Autodesk Inventor part; units mm, degrees
ref_plane "YZ Plane" through (0, 0, 0) normal (1, 0, 0) x (0, 1, 0)
ref_plane "XZ Plane" through (0, 0, 0) normal (0, 1, 0) x (-1, 0, 0)
ref_plane "XY Plane" through (0, 0, 0) normal (0, 0, 1) x (1, 0, 0)
sketch "Эскиз1" plane through (0, 0, 0) normal (0, 0, 1) x (1, 0, 0)
  circle A0 centre (0, 0) radius 40
  circle A1 centre (35, 35) radius 2
  circle A2 centre (-35, 35) radius 2
  circle A3 centre (-35, -35) radius 2
  circle A4 centre (35, -35) radius 2
  line L0 (72.777, 200) -> (-80, 200)
  line L1 (-80, 200) -> (-80, -200)
  line L2 (-80, -200) -> (72.777, -200)
  line L3 (72.777, -200) -> (72.777, 200)
  point P0 (0, 0)
  dimension "d0" = 400
  dimension "d1" = 200
  dimension "d2" = 80
extrude "Выдавливание1" add sketch "Эскиз1" along normal blind 4
sketch "Эскиз3" plane through (0, 0, 4) normal (0, 0, 1) x (1, 0, 0)
  line L0 (72.777, 200) -> (62.777, 200)
  line L1 (62.777, 200) -> (62.777, 196)
  line L2 (62.777, 196) -> (72.777, 196)
  line L3 (72.777, 196) -> (72.777, 200)
  line L4 (72.777, 200) -> (-80, 200)
  line L5 (52.777, 200) -> (42.777, 200)
  line L6 (42.777, 200) -> (42.777, 196)
  line L7 (42.777, 196) -> (52.777, 196)
  line L8 (52.777, 196) -> (52.777, 200)
  line L9 (32.777, 200) -> (22.777, 200)
  line L10 (22.777, 200) -> (22.777, 196)
  line L11 (22.777, 196) -> (32.777, 196)
  line L12 (32.777, 196) -> (32.777, 200)
  line L13 (12.777, 200) -> (2.777, 200)
  line L14 (2.777, 200) -> (2.777, 196)
  line L15 (2.777, 196) -> (12.777, 196)
  line L16 (12.777, 196) -> (12.777, 200)
  line L17 (-7.223, 200) -> (-17.223, 200)
  line L18 (-17.223, 200) -> (-17.223, 196)
  line L19 (-17.223, 196) -> (-7.223, 196)
  line L20 (-7.223, 196) -> (-7.223, 200)
  line L21 (-27.223, 200) -> (-37.223, 200)
  line L22 (-37.223, 200) -> (-37.223, 196)
  line L23 (-37.223, 196) -> (-27.223, 196)
  line L24 (-27.223, 196) -> (-27.223, 200)
  line L25 (-47.223, 200) -> (-57.223, 200)
  line L26 (-57.223, 200) -> (-57.223, 196)
  line L27 (-57.223, 196) -> (-47.223, 196)
  line L28 (-47.223, 196) -> (-47.223, 200)
  line L29 (-67.223, 200) -> (-77.223, 200)
  line L30 (-77.223, 200) -> (-77.223, 196)
  line L31 (-77.223, 196) -> (-67.223, 196)
  line L32 (-67.223, 196) -> (-67.223, 200)
  line L33 (0, 0) -> (123.2904, 0) construction
  line L34 (72.777, -200) -> (62.777, -200)
  line L35 (62.777, -200) -> (62.777, -196)
  line L36 (62.777, -196) -> (72.777, -196)
  line L37 (72.777, -196) -> (72.777, -200)
  line L38 (72.777, -200) -> (-80, -200)
  line L39 (52.777, -200) -> (42.777, -200)
  line L40 (42.777, -200) -> (42.777, -196)
  line L41 (42.777, -196) -> (52.777, -196)
  line L42 (52.777, -196) -> (52.777, -200)
  line L43 (32.777, -200) -> (22.777, -200)
  line L44 (22.777, -200) -> (22.777, -196)
  line L45 (22.777, -196) -> (32.777, -196)
  line L46 (32.777, -196) -> (32.777, -200)
  line L47 (12.777, -200) -> (2.777, -200)
  line L48 (2.777, -200) -> (2.777, -196)
  line L49 (2.777, -196) -> (12.777, -196)
  line L50 (12.777, -196) -> (12.777, -200)
  line L51 (-7.223, -200) -> (-17.223, -200)
  line L52 (-17.223, -200) -> (-17.223, -196)
  line L53 (-17.223, -196) -> (-7.223, -196)
  line L54 (-7.223, -196) -> (-7.223, -200)
  line L55 (-27.223, -200) -> (-37.223, -200)
  line L56 (-37.223, -200) -> (-37.223, -196)
  line L57 (-37.223, -196) -> (-27.223, -196)
  line L58 (-27.223, -196) -> (-27.223, -200)
  line L59 (-47.223, -200) -> (-57.223, -200)
  line L60 (-57.223, -200) -> (-57.223, -196)
  line L61 (-57.223, -196) -> (-47.223, -196)
  line L62 (-47.223, -196) -> (-47.223, -200)
  line L63 (-67.223, -200) -> (-77.223, -200)
  line L64 (-77.223, -200) -> (-77.223, -196)
  line L65 (-77.223, -196) -> (-67.223, -196)
  line L66 (-67.223, -196) -> (-67.223, -200)
  point P0 (-87.223, 200)
  point P1 (-87.223, -200)
  dimension "d7" = 10
  dimension "d8" = 4
  dimension "d11" = 20
extrude "Выдавливание2" cut sketch "Эскиз3" against normal blind 4
properties part number "задняя стенка"
Source: CAD feature listing. Evaluate the final solid. Frame: model axes, mm. Round coordinates to 2 decimals unless told otherwise and drop trailing zeros. Order: outer loops, then holes, each group sorted by start corner. A loop starts at its lowest first (then second) coordinate and runs counter-clockwise, first axis right, second up. Notation, with made-up numbers: (89, 4) -> (145, 4) arc R19 ccw to (145, 23) -> close; hole circle Ø7 at (-25, 70.5). An arc over 180 degrees is marked (long way). One line per item, written item: value. Start each with the question number.
Q1. Material intervals for probe 1 along Y at (x, z) = (0, 2); probe 2 along Y at (x, z) = (-35, 2.35); probe 3 along Y at (x, z) = (-72.5, 0.7), sorted ascending.
Q2. Pin query (flat end, axial travel): pin 1 (2 mm diameter, centred on x = -13.5, z = 2.5, fed in from +Y); pin 2 (1.2 mm diameter, centred on y = -198.5, z = 2, fed in from +X); pin 3 (1.2 mm diameter, centred on x = -52, z = 2.5, fed in from -Y). Return the tip coordinate at first contact, or that it passes through.
Q3. Draft query along Y for faces 1 (the cylindrical face through (-8.67, 39.05, 1.97)), 2 (the flat face through (-5, 47, 4)). Return one class per face: pulls with the +Y half, pulls with the -Y half, needs draft (parallel to the pull), parting line crosses it, or undercut.
Q4. Section query C-C (x = 46.5). Return the cut outline in (y, z).
Q5. Section query A-A (x = 8). Return the cut outline in (y, z).
Q6. Section query B-B (z = 2.05). Give the number of separate pieces and of enclosed holes in the cut face, plus the area to 3 significant figures.
Findings below:
1. probe 1: -200 to -40, 40 to 200
1. probe 2: -196 to -37, -33 to -19.36, 19.36 to 33, 37 to 196
1. probe 3: -196 to 196
2. pin 1: y = 196
2. pin 2: x = 62.78
2. pin 3: y = -196
3. face 1: undercut
3. face 2: needs draft
4. outline: (-196, 0) -> (196, 0) -> (196, 4) -> (-196, 4) -> close
5. outline: (-196, 0) -> (-39.19, 0) -> (-39.19, 4) -> (-196, 4) -> close; (39.19, 0) -> (196, 0) -> (196, 4) -> (39.19, 4) -> close
6. separate pieces: 1
6. enclosed holes: 5
6. area: 55,400 mm²
